Here's how the part is built. I have some questions about the finished solid (model axes, mm). A direction names the side the tool comes from. Round coordinates to 2 decimals unless told otherwise and drop trailing zeros. Order: outer loops, then holes, each group sorted by start corner. A loop starts at its lowest first (then second) coordinate and runs counter-clockwise, first axis right, second up. Notation, with made-up numbers: (-36.75, 54) - (0.25, 54) arc R23 ccw to (0.25, 62) - close; hole circle Ø1 at (-33.5, -36). An arc over 180 degrees is marked (long way). Answer as a JSON object with one key per item and string values.
```python
from build123d import *

# Parameters (mm, degrees)
F0_W     = 53.1
F0_H     = 24.8
F1_DEPTH = 13
F2_R     = 1
F3_W     = 50.7
F3_H     = 22.4
F4_DEPTH = 10


with BuildPart() as f1:
    # F0 (on Top) → F1 (new body)
    with BuildSketch(Plane.XY):
        with Locations((26.55, 12.4)):
            Rectangle(F0_W, F0_H)
    extrude(amount=F1_DEPTH)

    # F2
    f2_edges = [f1.edges().sort_by_distance(p)[0] for p in [
        (53.1, 24.8, 6.5),
        (53.1, 0, 6.5),
        (0, 24.8, 6.5),
        (0, 0, 6.5),
    ]]
    fillet(f2_edges, radius=F2_R)

    # F3 (on face) → F4 (cut)
    with BuildSketch(Plane.XY.offset(13)):
        with Locations((26.55, 12.4)):
            Rectangle(F3_W, F3_H)
    extrude(amount=-F4_DEPTH, mode=Mode.SUBTRACT)


solid = f1.part
```
1. For P1, Ø12, axis at x = 13, y = 15.5, coming from the +Z side; P2, Ø4, axis at x = 15, y = 6.5, coming from the -Z side, each with a flat end and sliding along its axis, tell me the tip position at first contact or that it passes through.
Responses:
{"P1": "z = 3", "P2": "z = 0"}
2. Imagine slicing it at A-A (z = 5.5). List the corners of the cut face in (x, y) for me.
Responses:
{"outline": "(0, 1) arc R1 ccw to (1, 0) - (52.1, 0) arc R1 ccw to (53.1, 1) - (53.1, 23.8) arc R1 ccw to (52.1, 24.8) - (1, 24.8) arc R1 ccw to (0, 23.8) - close; hole (1.2, 1.2) - (51.9, 1.2) - (51.9, 23.6) - (1.2, 23.6) - close"}
3. Thinking about a two-plate mould opening in X: for faces 3 (the face through (0, 12, 6)), 4 (the face through (53.1, 12, 6)), 5 (the face through (26, 1.2, 8)), which applies, pulls with the +X half, pulls with the -X half, needs draft (parallel to the pull), parting line crosses it, or undercut?
Responses:
{"face 3": "pulls with the -X half", "face 4": "pulls with the +X half", "face 5": "undercut"}
4. For faces 1 (the face through (0.285, 0.301, 6.591)), 2 (the face through (51.9, 12, 8)), which set-ups out of +Z, -Z, +X, -X, +Y, -Y let a thin tool reach every point of the face, with its end or its side?
Responses:
{"face 1": "+Z, -Z, -X, -Y", "face 2": "+Z"}
5. If I drill on L1, parallel to X at y = 16.25, z = 4.5; L2, parallel to Y at x = 16.5, z = 8.5; L3, parallel to Z at x = 10, y = 11.25, over which ranges is the centre line in solid material (lowest first)? Write a range as [from, to].
Responses:
{"L1": "[0, 1.2], [51.9, 53.1]", "L2": "[0, 1.2], [23.6, 24.8]", "L3": "[0, 3]"}
6. Imagine slicing it at B-B (y = 22.5). List the corners of the cut face in (x, z) for me.
Responses:
{"outline": "(0, 0) - (53.1, 0) - (53.1, 13) - (51.9, 13) - (51.9, 3) - (1.2, 3) - (1.2, 13) - (0, 13) - close"}
7. Imagine slicing it at C-C (x = 37). List the corners of the cut face in (y, z) for me.
Responses:
{"outline": "(0, 0) - (24.8, 0) - (24.8, 13) - (23.6, 13) - (23.6, 3) - (1.2, 3) - (1.2, 13) - (0, 13) - close"}
